Source: CAD feature listing. Evaluate the final solid. Frame: model axes, mm. A direction names the side the tool comes from. Round coordinates to 2 decimals unless told otherwise and drop trailing zeros. Order: outer loops, then holes, each group sorted by start corner. A loop starts at its lowest first (then second) coordinate and runs counter-clockwise, first axis right, second up. Notation, with made-up numbers: (41.25, -19.5) - (88.25, -19.5) arc R24 cw to (88.25, 4.5) - close; hole circle Ø6 at (67.5, 7). An arc over 180 degrees is marked (long way). Return JSON: item names as keys, results as strings. Group by question number.
1) Section B-B, the plane x = -34.5. Return loops of the section in (y, z), plus the area to 3 significant figures.
2) Mould query, pull axis Z, two halves, no side actions, for faces 4 (the flat face through (-20, 9, 23)), 5 (the flat face through (20, 4, 14)), 6 (the flat face through (-29, 8, 100)). Classes: pulls with the +Z half, pulls with the -Z half, needs draft (parallel to the pull), parting line crosses it, or undercut.
3) Ray query, line 1 (X direction, y = 12.9, z = 87); line 2 (X direction, y = 11.45, z = 87); line 3 (Z direction, x = -22.5, y = 2.75). Return the intervals inside material, ascending. Write a range as from..to.
4) Section A-A, the plane z = 64.5. Return loops of the section in (x, y).
5) Section C-C, the plane y = 1.75. Return loops of the section in (x, z).
6) Contact query for flat-ended pins moving along their axis: P1, Ø4, axis at y = 19.5, z = -23, coming from the -X side; P2, Ø3.5, axis at x = -21, y = 4.5, coming from the +Z side; P3, Ø8, axis at x = -22, z = 50, coming from the -Y side; P4, Ø4.5, axis at y = 9, z = -8, coming from the -X side. Output: stop coordinate, or through.
7) Access query for faces 1 (the flat face through (-22, 8, -24)), 2 (the flat face through (0, 5, 40)), 3 (the flat face through (2.5, 12, -27)). Directions: +Z, -Z, +X, -X, +Y, -Y. A direction counts if a zero-diameter tool reaches every point of the face in a straight line with its end or side. Return the directions, or none.
8) Section D-D, the plane z = 41. Return loops of the section in (x, y).
```python
from build123d import *

# Parameters (mm, degrees)
SKETCH1_W            = 40
SKETCH1_H            = 50
BOSS_EXTRUDE1_DEPTH  = 5
SKETCH3_W            = 5
SKETCH3_H            = 5
BOSS_EXTRUDE5_DEPTH  = 20
SKETCH3_3_W          = 15
SKETCH3_3_H          = 5
SKETCH3_3_W_2        = 5
BOSS_EXTRUDE6_DEPTH  = 10
CUT_EXTRUDE3_DEPTH   = 4
SKETCH11_W           = 5
SKETCH11_H           = 5
BOSS_EXTRUDE10_DEPTH = 5
SKETCH12_R           = 1.5
CUT_EXTRUDE4_DEPTH   = 5
SKETCH14_W           = 10
SKETCH14_H           = 5
SKETCH14_W_2         = 5
BOSS_EXTRUDE12_DEPTH = 30
SKETCH15_W           = 40
SKETCH15_H           = 15
BOSS_EXTRUDE13_DEPTH = 5
BOSS_EXTRUDE15_DEPTH = 16.5
BOSS_EXTRUDE17_DEPTH = 11.5
SKETCH18_W           = 5
SKETCH18_H           = 15
BOSS_EXTRUDE18_DEPTH = 40
BOSS_EXTRUDE19_DEPTH = 8
SKETCH20_W           = 6
SKETCH20_H           = 5
BOSS_EXTRUDE20_DEPTH = 6
SKETCH21_R           = 1.5
CUT_EXTRUDE5_DEPTH   = 5
SKETCH24_R           = 1.05
CUT_EXTRUDE7_DEPTH   = 5
BOSS_EXTRUDE21_START = 3
BOSS_EXTRUDE21_DEPTH = 3


with BuildPart() as part:
    # Sketch1 → Boss-Extrude1 (new body)
    with BuildSketch(Plane(origin=(0, 0, 0), x_dir=(1, 0, 0), z_dir=(0, 1, 0))):
        Rectangle(SKETCH1_W, SKETCH1_H)
    extrude(amount=BOSS_EXTRUDE1_DEPTH)

    # Sketch3 → Boss-Extrude5 (add)
    with BuildSketch(Plane(origin=(0, 5, 0), x_dir=(1, 0, 0), z_dir=(0, 1, 0))):
        with Locations((9, 22.5)):
            Rectangle(SKETCH3_W, SKETCH3_H)
    extrude(amount=BOSS_EXTRUDE5_DEPTH)

    # Sketch3_3 → Boss-Extrude6 (add)
    with BuildSketch(Plane(origin=(0, 5, 0), x_dir=(1, 0, 0), z_dir=(0, 1, 0))):
        with Locations((-1, 22.5)):
            Rectangle(SKETCH3_3_W, SKETCH3_3_H)
        Polygon((-16.5, -20), (-16.5, 25), (-20, 25), (-20, -25), (6.5, -25), (6.5, -20), align=None)
        with Locations((17.5, -22.5)):
            Rectangle(SKETCH3_3_W_2, SKETCH3_3_H)
    extrude(amount=BOSS_EXTRUDE6_DEPTH)

    # Sketch8 → Cut-Extrude3 (cut)
    with BuildSketch(Plane.ZY.offset(20)):
        with BuildLine():
            Line((1, 15), (-21, 15))
            ThreePointArc((-21, 15), (-10, 4), (1, 15))
        make_face()
    extrude(amount=-CUT_EXTRUDE3_DEPTH, mode=Mode.SUBTRACT)

    # Sketch11 → Boss-Extrude10 (add)
    with BuildSketch(Plane(origin=(0, 0, -25), x_dir=(-1, 0, 0), z_dir=(0, 0, -1))):
        with Locations((0, 12.5)):
            Rectangle(SKETCH11_W, SKETCH11_H)
    extrude(amount=BOSS_EXTRUDE10_DEPTH)

    # Sketch12 → Cut-Extrude4 (cut)
    with BuildSketch(Plane.XZ.offset(-10)):
        with Locations(Location((0, -27.5, 0), (0, 0, 270))):
            Circle(SKETCH12_R)
    extrude(amount=-CUT_EXTRUDE4_DEPTH, mode=Mode.SUBTRACT)

    # Sketch14 → Boss-Extrude12 (add)
    with BuildSketch(Plane.XY.offset(25)):
        with Locations((0, 2.5)):
            Rectangle(SKETCH14_W, SKETCH14_H)
        with Locations((-17.5, 12.5)):
            Rectangle(SKETCH14_W_2, SKETCH14_H)
        with Locations((17.5, 12.5)):
            Rectangle(SKETCH14_W_2, SKETCH14_H)
    extrude(amount=BOSS_EXTRUDE12_DEPTH)

    # Sketch15 → Boss-Extrude13 (add)
    with BuildSketch(Plane.XY.offset(55)):
        with Locations((0, 7.5)):
            Rectangle(SKETCH15_W, SKETCH15_H)
    extrude(amount=BOSS_EXTRUDE13_DEPTH)

    # Sketch16 → Boss-Extrude15 (add)
    with BuildSketch(Plane(origin=(20, 0, 0), x_dir=(0, 0, -1), z_dir=(1, 0, 0))):
        Polygon((-60, 0), (-55, 0), (-55, 10), (-55, 15), (-60, 15), align=None)
    extrude(amount=BOSS_EXTRUDE15_DEPTH)

    # Sketch17 → Boss-Extrude17 (add)
    with BuildSketch(Plane.ZY.offset(20)):
        Polygon((55, 0), (60, 0), (60, 15), (55, 15), (55, 10), align=None)
    extrude(amount=BOSS_EXTRUDE17_DEPTH)

    # Sketch18 → Boss-Extrude18 (add)
    with BuildSketch(Plane.XY.offset(60)):
        with Locations((34, 7.5)):
            Rectangle(SKETCH18_W, SKETCH18_H)
        with Locations((-29, 7.5)):
            Rectangle(SKETCH18_W, SKETCH18_H)
    extrude(amount=BOSS_EXTRUDE18_DEPTH)

    # Sketch19 → Boss-Extrude19 (add)
    with BuildSketch(Plane(origin=(-26.5, 0, 0), x_dir=(0, 0, -1), z_dir=(1, 0, 0))):
        with BuildLine():
            Line((-86.25, 15), (-93.75, 15))
            ThreePointArc((-93.75, 15), (-90, 11.25), (-86.25, 15))
        make_face()
    extrude(amount=BOSS_EXTRUDE19_DEPTH)

    # Sketch20 → Boss-Extrude20 (add)
    with BuildSketch(Plane.ZY.offset(31.5)):
        with Locations((87, 12.5)):
            Rectangle(SKETCH20_W, SKETCH20_H)
    extrude(amount=BOSS_EXTRUDE20_DEPTH)

    # Sketch21 → Cut-Extrude5 (cut)
    with BuildSketch(Plane.XZ.offset(-10)):
        with Locations(Location((-34.5, 87, 0), (0, 0, 270))):
            Circle(SKETCH21_R)
    extrude(amount=-CUT_EXTRUDE5_DEPTH, mode=Mode.SUBTRACT)

    # Sketch24 → Cut-Extrude7 (cut)
    with BuildSketch(Plane.ZY.offset(-31.5)):
        with Locations((93.5, 8)):
            Circle(SKETCH24_R)
        with Locations((86.5, 8)):
            Circle(SKETCH24_R)
    extrude(amount=-CUT_EXTRUDE7_DEPTH, mode=Mode.SUBTRACT)

    # Sketch25 → Boss-Extrude21 (add)
    with BuildSketch(Plane.ZY.offset(20).offset(BOSS_EXTRUDE21_START)):
        with BuildLine():
            Line((-21, 15), (-24, 15))
            Line((-24, 15), (-24, 0))
            Line((-24, 0), (4, 0))
            Line((4, 0), (4, 15))
            Line((4, 15), (1, 15))
            ThreePointArc((1, 15), (-10, 4), (-21, 15))
        make_face()
    extrude(amount=-BOSS_EXTRUDE21_DEPTH)


solid = part.part
```
Geometry check:
{
 "1": {"outline": "(10, 84) - (15, 84) - (15, 85.5) - (10, 85.5) - close; (10, 88.5) - (15, 88.5) - (15, 90) - (10, 90) - close", "area": "15.0 mm2"},
 "2": {"face 4": "undercut", "face 5": "needs draft", "face 6": "pulls with the +Z half"},
 "3": {"line 1": "-37.5..-36, -33..-18.5, 31.5..36.5", "line 2": "-37.5..-36, -33..-26.5, 31.5..36.5", "line 3": "-24..4, 55..60"},
 "4": {"outline": "(-31.5, 0) - (-26.5, 0) - (-26.5, 15) - (-31.5, 15) - close; (31.5, 0) - (36.5, 0) - (36.5, 15) - (31.5, 15) - close"},
 "5": {"outline": "(-31.5, 55) - (-5, 55) - (-5, 25) - (-20, 25) - (-20, 4) - (-23, 4) - (-23, -24) - (-20, -24) - (-20, -25) - (20, -25) - (20, 25) - (5, 25) - (5, 55) - (36.5, 55) - (36.5, 100) - (31.5, 100) - (31.5, 60) - (-26.5, 60) - (-26.5, 100) - (-31.5, 100) - close"},
 "6": {"P1": "x = 6.5", "P2": "z = 60", "P3": "y = 10", "P4": "through"},
 "7": {"face 1": "-Z, -X, +Y, -Y", "face 2": "+X, -X, +Y", "face 3": "-Z, +X, +Y, -Y"},
 "8": {"outline": "(-20, 10) - (-15, 10) - (-15, 15) - (-20, 15) - close; (-5, 0) - (5, 0) - (5, 5) - (-5, 5) - close; (15, 10) - (20, 10) - (20, 15) - (15, 15) - close"}
}
